from build123d import *

# Parameters (mm, degrees)
ESQUISSE1_W             = 10
ESQUISSE1_H             = 10
BOSS_EXTRU_1_DEPTH      = 3
ESQUISSE2_R             = 3.5
BOSS_EXTRU_2_DEPTH      = 3
ESQUISSE5_R             = 1.5
BOSS_EXTRU_4_DEPTH      = 7
BOSS_EXTRU_5_DEPTH      = 1
ENL_V_MAT_EXTRU_1_DEPTH = 5
CONG_1_R                = 1
CONG_5_R                = 0.5


with BuildPart() as part:
    # Esquisse1 → Boss.-Extru.1 (new body)
    with BuildSketch(Plane.XY):
        Rectangle(ESQUISSE1_W, ESQUISSE1_H)
    extrude(amount=BOSS_EXTRU_1_DEPTH)

    # Esquisse2 → Boss.-Extru.2 (add)
    with BuildSketch(Plane.XY.offset(3)):
        with Locations(Location((0, 0, 0), (0, 0, 180))):
            Circle(ESQUISSE2_R)
    extrude(amount=BOSS_EXTRU_2_DEPTH)

    # Esquisse5 → Boss.-Extru.4 (add)
    with BuildSketch(Plane.XY.offset(6)):
        Circle(ESQUISSE5_R)
    extrude(amount=BOSS_EXTRU_4_DEPTH)

    # Esquisse6 → Boss.-Extru.5 (add)
    with BuildSketch(Plane.XY.offset(13)):
        with BuildLine():
            Line((-0.710860958, -1), (-0.710860958, 1))
            ThreePointArc((-0.710860958, 1), (0, 1.710860958), (0.710860958, 1))
            Line((0.710860958, 1), (0.710860958, -1))
            ThreePointArc((0.710860958, -1), (0, -1.710860958), (-0.710860958, -1))
        make_face()
    extrude(amount=-BOSS_EXTRU_5_DEPTH)

    # Esquisse7 → Enlèv. mat.-Extru.1 (cut)
    with BuildSketch(Plane.XY.offset(13)):
        with BuildLine():
            Line((1.624079267, -0.75), (-1.624079267, -0.75))
            ThreePointArc((-1.624079267, -0.75), (-2.374079267, 0), (-1.624079267, 0.75))
            Line((-1.624079267, 0.75), (1.624079267, 0.75))
            ThreePointArc((1.624079267, 0.75), (2.374079267, 0), (1.624079267, -0.75))
        make_face()
    extrude(amount=-ENL_V_MAT_EXTRU_1_DEPTH, mode=Mode.SUBTRACT)

    # Congé1
    # the kernel refuses this fillet: 1 mm, written as the material it takes off along each edge
    with BuildSketch(Plane(origin=(-3.799038106, 0.75, 13), x_dir=(0, 0, -1), z_dir=(1, 0, 0)), Plane(origin=(3.799038106, -0.75, 13), x_dir=(0, 0, -1), z_dir=(-1, 0, 0))) as cong_1_piece_1:
        with BuildLine():
            CenterArc((CONG_1_R, CONG_1_R), CONG_1_R, 180, 90)
            Line((0, CONG_1_R), (0, 0))
            Line((0, 0), (CONG_1_R, 0))
        make_face()
    extrude(amount=7.598076211, mode=Mode.SUBTRACT)

    # Congé5
    cong_5_edges = [part.edges().sort_by_distance(p)[0] for p in [
        (3.5, 0, 3),
        (3.5, 0, 6),
    ]]
    fillet(cong_5_edges, radius=CONG_5_R)


solid = part.part
CAD build for the part. Positions are in the model's coordinates, mm. A direction names the side the tool comes from. Coordinates: 2 decimals unless noted, no trailing zeros. Write each loop counter-clockwise with the first axis right and the second up, starting at its lowest first coordinate (ties: lowest second). Pieces come first, ordered by that corner, then holes. Notation, with made-up numbers: M -29,63.25 L -18,63.25 A36 ccw -18,97.25 Z; hole C 54.5,19.25 d4. An arc over 180 degrees is marked long. Answer as a JSON object with one key per item and string values. Group by question number.
1) Tool access for faces 4 (the face through (-1.2, -0.9, 8.6)), 5 (the face through (-3.233, 1.341, 4.486)), 6 (the face through (-0.01, 1.71, 12.51)), 7 (the face through (0, 0.75, 10)): list every direction of +Z, -Z, +X, -X, +Y, -Y with a clear straight run to the whole face (end or side of a thin tool).
2) Saw through at A-A (y = 0). Write the cut outline in (x, z), plus the area to 3 significant figures.
3) Mould opens along Y. For faces 1 (the face through (0.01, -1.71, 12.51)), 2 (the face through (-4.5, 0.1, 3)), 3 (the face through (-0.02, 0.93, 12.57)) say: +Y half, -Y half, draft (parallel to the pull), parting line (faces both ways), or undercut.
4) Saw through at B-B (x = 0). Write the cut outline in (y, z).
5) Pin check, flat tips, straight feed: pin 1 Ø2 at (y, z) = (-2.5, 5) entering from +X; pin 2 Ø1.3 at (x, z) = (0, 10) entering from +Y; pin 3 Ø3 at (y, z) = (1, 11.5) entering from +X. Stop position of each tip, or through.
6) Saw through at C-C (z = 6.25). Write the cut outline in (x, y).
7) Saw through at D-D (x = 4.75). Write the cut outline in (y, z), plus the area to 3 significant figures.
8) Wall check: line 1 (Z direction, x = 1, y = -4); line 2 (Y direction, x = 0.5, z = 8.75); line 3 (X direction, y = -0.75, z = 7). Give the ranges that are in metal, low to high. Write a range as from..to.
Values follow:
{
 "1": {"face 4": "none", "face 5": "+Z", "face 6": "+Z, +Y", "face 7": "+Z, +X, -X"},
 "2": {"outline": "M -5,0 L 5,0 L 5,3 L 4,3 A0.5 cw 3.5,3.5 L 3.5,5.5 A0.5 ccw 3,6 L 1.5,6 L 1.5,8 L -1.5,8 L -1.5,6 L -3,6 A0.5 ccw -3.5,5.5 L -3.5,3.5 A0.5 cw -4,3 L -5,3 Z", "area": "57.0 mm2"},
 "3": {"face 1": "-Y half", "face 2": "draft", "face 3": "undercut"},
 "4": {"outline": "M -5,0 L 5,0 L 5,3 L 4,3 A0.5 cw 3.5,3.5 L 3.5,5.5 A0.5 ccw 3,6 L 1.5,6 L 1.5,12 L 1.71,12 L 1.71,13 A1 ccw 0.75,12 L 0.75,8 L -0.75,8 L -0.75,12 A1 ccw -1.71,13 L -1.71,12 L -1.5,12 L -1.5,6 L -3,6 A0.5 ccw -3.5,5.5 L -3.5,3.5 A0.5 cw -4,3 L -5,3 Z"},
 "5": {"pin 1": "stops at x = 3.16", "pin 2": "stops at y = 1.5", "pin 3": "stops at x = 1.3"},
 "6": {"outline": "C 0,0 d3"},
 "7": {"outline": "M -5,0 L 5,0 L 5,3 L -5,3 Z", "area": "30.0 mm2"},
 "8": {"line 1": "z = 0..3", "line 2": "y = -1.41..-0.75, 0.75..1.41", "line 3": "x = -1.3..1.3"}
}
